Geometry: final body of the model. Coordinates: model frame, mm. A direction names the side the tool comes from. Round coordinates to 2 decimals unless told otherwise and drop trailing zeros. Loops run counter-clockwise (first coordinate to the right, second up) from the corner with the lowest first, then second, coordinate; pieces in that order, holes last. Notation, with made-up numbers: (12, 79) -> (30, 79) arc R8 cw to (30, 92) -> close; hole circle Ø11 at (80.5, -26). An arc over 180 degrees is marked (long way). Answer in a Markdown table with one row per item.
```python
from build123d import *

# Parameters (mm, degrees)
SKETCH3_W           = 38.1
SKETCH3_H           = 38.1
SKETCH4_R           = 10
CUT_EXTRUDE1_DEPTH  = 917.183483622
SKETCH5_R           = 30
SKETCH5_R_2         = 10
BOSS_EXTRUDE1_DEPTH = 38.1
FILLET1_R           = 38.1
SKETCH6_W           = 7.62
SKETCH6_H           = 80.541178389
CUT_EXTRUDE2_DEPTH  = 60


with BuildPart() as part:
    # Sweep1: sweep along a path in Sketch1
    with BuildLine(Plane(origin=(0, 0, 0), x_dir=(0, 0, -1), z_dir=(1, 0, 0))) as sweep1_path:
        Line((0, 0), (0, 91.466893968))
        Line((0, 91.466893968), (250, 225))
        Line((250, 225), (842.350315886, -91.393510157))
        ThreePointArc((842.350315886, -91.393510157), (857.076574448, -105.407871929), (862.5, -125))
    # Sketch3 → Sweep1 (sweep)
    with BuildSketch(Plane(origin=(0, 0, 0), x_dir=(1, 0, 0), z_dir=(0, 1, 0))):
        Rectangle(SKETCH3_W, SKETCH3_H)
    sweep(path=sweep1_path.line, transition=Transition.RIGHT)

    # Sketch4 → Cut-Extrude1 (cut, through all)
    with BuildSketch(Plane(origin=(19.05, 0, 0), x_dir=(0, 0, -1), z_dir=(1, 0, 0))):
        Circle(SKETCH4_R)
        with Locations((250, 225)):
            Circle(SKETCH4_R)
    extrude(amount=-CUT_EXTRUDE1_DEPTH, mode=Mode.SUBTRACT)

    # Sketch5 → Boss-Extrude1 (add)
    # profile 1 of 2: a face of its own
    with BuildSketch(Plane(origin=(19.05, 0, 0), x_dir=(0, 0, -1), z_dir=(1, 0, 0))):
        Circle(SKETCH5_R)
        Circle(SKETCH5_R_2, mode=Mode.SUBTRACT)
    # profile 2 of 2: a face of its own
    with BuildSketch(Plane(origin=(19.05, 0, 0), x_dir=(0, 0, -1), z_dir=(1, 0, 0))):
        with Locations((250, 225)):
            Circle(SKETCH5_R)
        with Locations((250, 225)):
            Circle(SKETCH5_R_2, mode=Mode.SUBTRACT)
    extrude(amount=-BOSS_EXTRUDE1_DEPTH)

    # Fillet1
    fillet1_edges = [part.edges().sort_by_distance(p)[0] for p in [
        (0, 230.884475737, -279.417221917),
        (0, 197.277985894, -261.46690603),
        (0, 80.044948857, -19.05),
        (0, 102.888839079, 19.05),
        (0, 23.175364075, 19.05),
        (0, 23.175364075, -19.05),
        (0, 230.884475737, -220.582778083),
        (0, 197.277985894, -238.53309397),
    ]]
    fillet(fillet1_edges, radius=FILLET1_R)

    # Sketch6 → Cut-Extrude2 (cut)
    with BuildSketch(Plane(origin=(0, -30, 0), x_dir=(-1, 0, 0), z_dir=(0, -1, 0))):
        with Locations((-15.24, -3.428675544)):
            Rectangle(SKETCH6_W, SKETCH6_H)
        with Locations((0, -3.428675544)):
            Rectangle(SKETCH6_W, SKETCH6_H)
        with Locations((15.24, -3.428675544)):
            Rectangle(SKETCH6_W, SKETCH6_H)
    extrude(amount=-CUT_EXTRUDE2_DEPTH, mode=Mode.SUBTRACT)


solid = part.part
```
Item 1: Reachability of faces 1 (the face through (-0.3, 76.5, -24.3)), 2 (the face through (-3.81, 13, 0)), 3 (the face through (11.43, 13, 0)), 4 (the face through (0.267, 141.478, -134.064)) from +Z, -Z, +X, -X, +Y, -Y: full face, straight path, thin tool, end or side. Return the list, or none.
Answer:
| item | result |
|---|---|
| face 1 | +X, -X |
| face 2 | +Z, -Y |
| face 3 | +Z, +X, -Y |
| face 4 | +X, -X, -Y |
Item 2: Draft query along Z for faces 5 (the face through (0, 47, -19.05)), 6 (the face through (0.27, -95.24, -873.19)), 7 (the face through (-0.27, 169.78, -106.18)), 8 (the face through (0, 255, -250)). Return one class per face: pulls with the +Z half, pulls with the -Z half, needs draft (parallel to the pull), parting line crosses it, or undercut.
Answer:
| item | result |
|---|---|
| face 5 | undercut |
| face 6 | pulls with the -Z half |
| face 7 | pulls with the +Z half |
| face 8 | parting line crosses it |
Item 3: Line query: probe 1 along Z at (x, y) = (14, 75.5); probe 2 along Z at (x, y) = (9.5, 109); probe 3 along Y at (x, z) = (-6, 0). Output: solid intervals per line, ascending. Write a range as [from, to].
Answer:
| item | result |
|---|---|
| probe 1 | z = [-570.33, -489.46], [-23.73, 19.05] |
| probe 2 | z = [-507.61, -426.74], [-73.26, 5.71] |
| probe 3 | y = [-30, -10], [10, 113.04] |
Item 4: Cut plane B-B (y = 0). Output: boundary loops of the cut face in (x, z).
Answer:
| item | result |
|---|---|
| outline | (-19.05, -711.68) -> (19.05, -711.68) -> (19.05, -630.81) -> (-19.05, -630.81) -> close; (-11.43, -30) -> (-3.81, -30) -> (-3.81, -10) -> (-11.43, -10) -> close; (-11.43, 10) -> (-3.81, 10) -> (-3.81, 30) -> (-11.43, 30) -> close; (3.81, -30) -> (11.43, -30) -> (11.43, -10) -> (3.81, -10) -> close; (3.81, 10) -> (11.43, 10) -> (11.43, 30) -> (3.81, 30) -> close |
Item 5: Cut plane D-D (y = -60.5). Output: boundary loops of the cut face in (x, z), then the cut area to 3 significant figures.
Answer:
| item | result |
|---|---|
| outline | (-19.05, -824.95) -> (19.05, -824.95) -> (19.05, -744.08) -> (-19.05, -744.08) -> close |
| area | 3,080 mm² |
Item 6: Pin query (flat end, axial travel): pin 1 Ø2.5 at (x, z) = (15, 9) entering from -Y; pin 2 Ø5 at (x, y) = (14.5, -85) entering from -Z; pin 3 Ø10 at (x, z) = (8, -103.5) entering from +Y. Return the tip coordinate at first contact, or that it passes through.
Answer:
| item | result |
|---|---|
| pin 1 | stops at y = 30 |
| pin 2 | stops at z = -867.53 |
| pin 3 | stops at y = 171.02 |
Item 7: Cut plane C-C (z = -671). Output: boundary loops of the cut face in (x, y).
Answer:
| item | result |
|---|---|
| outline | (-19.05, -21.47) -> (19.05, -21.47) -> (19.05, 21.73) -> (-19.05, 21.73) -> close |
Item 8: Cut plane A-A (y = 125.5). Output: boundary loops of the cut face in (x, z), then the cut area to 3 significant figures.
Answer:
| item | result |
|---|---|
| outline | (-19.05, -476.72) -> (19.05, -476.72) -> (19.05, -395.85) -> (-19.05, -395.85) -> close; (-19.05, -104.15) -> (19.05, -104.15) -> (19.05, -23.28) -> (-19.05, -23.28) -> close |
| area | 6,160 mm² |
